CAD build for the part. Positions are in the model's coordinates, mm. A direction names the side the tool comes from. Give positions to 0.01 mm unless a question says otherwise; leave off trailing zeros. Write each loop counter-clockwise with the first axis right and the second up, starting at its lowest first coordinate (ties: lowest second). Pieces come first, ordered by that corner, then holes. Notation, with made-up numbers: (42.5, 10) - (98.5, 10) arc R30 cw to (98.5, 49) - close; hole circle Ø11 at (8, 60.25). An arc over 180 degrees is marked (long way). Answer as a JSON object with one key per item and string values.
from build123d import *

# Parameters (mm, degrees)
F0_R     = 7.95
F2_DEPTH = 3
F4_R     = 8.75
F4_R_2   = 7.95
F5_DEPTH = 1.5
F3_R     = 7.302196
F6_DEPTH = 1.5


with BuildPart() as f2:
    # F0 (on Top) → F2 (new body)
    with BuildSketch(Plane.XY):
        Circle(F0_R)
    extrude(amount=F2_DEPTH)

    # F4 (on face) → F5 (join, symmetric)
    with BuildSketch(Plane.XY.offset(3)):
        Circle(F4_R)
        Circle(F4_R_2, mode=Mode.SUBTRACT)
    extrude(amount=F5_DEPTH, both=True)

    # F3 (on Top) → F6 (join, symmetric)
    with BuildSketch(Plane.XY):
        Circle(F3_R)
    extrude(amount=F6_DEPTH, both=True)


solid = f2.part
Item 1: Flat gauge pin, fed straight in: P1, Ø2, axis at y = 6, z = 1, coming from the +X side. Where does the tip first touch, or does it go through?
Entries:
{"P1": "x = 7.09"}
Item 2: Mould opens along Y. For faces 4 (the cylindrical face through (6.745, -2.797, -0.74)), 5 (the flat face through (0, 0, 3)), 6 (the flat face through (2, -8, 1.5)) say: +Y half, -Y half, draft (parallel to the pull), parting line (faces both ways), or undercut.
Entries:
{"face 4": "parting line", "face 5": "undercut", "face 6": "draft"}
Item 3: Cut at C-C (z = 2.75). Give the cut face in (x, y), and give its area (3 significant figures).
Entries:
{"outline": "circle Ø17.5 at (0, 0)", "area": "241 mm2"}
Item 4: Cut at D-D (z = 3.65). Give the cut face in (x, y), and give its area (3 significant figures).
Entries:
{"outline": "circle Ø17.5 at (0, 0); hole circle Ø15.9 at (0, 0)", "area": "42.0 mm2"}
Item 5: Which spindle directions (+Z, -Z, +X, -X, +Y, -Y) get a long thin tool onto all of the face, cutting with end or side? Do faces 1 (the cylindrical face through (-6.944, -5.324, 3.021)), 2 (the cylindrical face through (-1.72, -7.76, 0.74)), 3 (the cylindrical face through (-1.72, -7.76, 3.74)). Say none if no direction does.
Entries:
{"face 1": "+Z, -Z", "face 2": "-Z", "face 3": "+Z"}
Item 6: Probe line 1 (Y direction, x = 0, z = 4.1); line 2 (Z direction, x = -6, y = 3.75); line 3 (X direction, y = 2, z = 3.25). List the from-to ranges inside material, lowest first. Write a range as from..to.
Entries:
{"line 1": "-8.75..-7.95, 7.95..8.75", "line 2": "-1.5..3", "line 3": "-8.52..-7.69, 7.69..8.52"}
Item 7: Cut at A-A (y = 0). Give the cut face in (x, z), and give its area (3 significant figures).
Entries:
{"outline": "(-8.75, 1.5) - (-7.95, 1.5) - (-7.95, 0) - (-7.3, 0) - (-7.3, -1.5) - (7.3, -1.5) - (7.3, 0) - (7.95, 0) - (7.95, 1.5) - (8.75, 1.5) - (8.75, 4.5) - (7.95, 4.5) - (7.95, 3) - (-7.95, 3) - (-7.95, 4.5) - (-8.75, 4.5) - close", "area": "74.4 mm2"}
